Verification items for the finished model (mm, model axes). A direction names the side the tool comes from. Round coordinates to 2 decimals unless told otherwise and drop trailing zeros. Order: outer loops, then holes, each group sorted by start corner. A loop starts at its lowest first (then second) coordinate and runs counter-clockwise, first axis right, second up. Notation, with made-up numbers: (4.25, -24.75) -> (47.25, -24.75) arc R15 cw to (47.25, 4.25) -> close; hole circle Ø5 at (72.25, 80.25). An arc over 180 degrees is marked (long way). Put each result on its own line as item: value.
```python
from build123d import *

# Parameters (mm, degrees)
BOSS_EXTRUDE1_DEPTH    = 105
SKETCH3_R              = 1.75
CUT_EXTRUDE1_DEPTH     = 15
CUT_EXTRUDE2_START     = -3
CUT_EXTRUDE2_OUTLINE_R = 1.75
CUT_EXTRUDE2_DEPTH     = 3
FILLET1_R              = 1


# Read off the part's stored shape, not the designer's step: Cut-Extrude2
with BuildPart() as part:
    # Sketch1 → Boss-Extrude1 (new body)
    with BuildSketch(Plane.XY):
        with BuildLine():
            ThreePointArc((-43.375, -14.309088021), (-30.875, -19), (-18.375, -14.309088021))
            Line((-18.375, -14.309088021), (-18.375, -3.570714214))
            ThreePointArc((-18.375, -3.570714214), (-30.875, -13), (-43.375, -3.570714214))
            Line((-43.375, -3.570714214), (-43.375, -14.309088021))
        make_face()
    extrude(amount=BOSS_EXTRUDE1_DEPTH)

    # Sketch3 → Cut-Extrude1 (cut)
    with BuildSketch(Plane(origin=(0, 0, 0), x_dir=(-1, 0, 0), z_dir=(0, 0, -1))):
        with Locations((22.271353455, -12.287280664)):
            Circle(SKETCH3_R)
        with Locations((30.875, -15)):
            Circle(SKETCH3_R)
        with Locations((39.478646545, -12.287280664)):
            Circle(SKETCH3_R)
    cut_extrude1 = extrude(amount=-CUT_EXTRUDE1_DEPTH, mode=Mode.SUBTRACT)

    # Cut-Extrude2 outline → Cut-Extrude2 (cut)
    # profile 1 of 3: a face of its own
    with BuildSketch(Plane(origin=(0, 0, 4), x_dir=(-1, 0, 0), z_dir=(0, 0, -1)).offset(CUT_EXTRUDE2_START)):
        with BuildLine():
            Line((20.383772748, -14.983025288), (23.662146428, -15.26984582))
            Line((23.662146428, -15.26984582), (25.93448352, -12.024612131))
            ThreePointArc((25.93448352, -12.024612131), (23.418506327, -10.648976576), (21.265316867, -8.755226444))
            Line((21.265316867, -8.755226444), (18.992979775, -12.000460133))
            Line((18.992979775, -12.000460133), (20.383772748, -14.983025288))
        make_face()
        with Locations((22.271353455, -12.287280664)):
            Circle(CUT_EXTRUDE2_OUTLINE_R, mode=Mode.SUBTRACT)
    # profile 2 of 3: a face of its own
    with BuildSketch(Plane(origin=(0, 0, 4), x_dir=(-1, 0, 0), z_dir=(0, 0, -1)).offset(CUT_EXTRUDE2_START)):
        with BuildLine():
            ThreePointArc((40.484683133, -8.755226444), (38.331493673, -10.648976576), (35.81551648, -12.024612131))
            Line((35.81551648, -12.024612131), (38.087853572, -15.26984582))
            Line((38.087853572, -15.26984582), (41.366227252, -14.983025288))
            Line((41.366227252, -14.983025288), (42.757020225, -12.000460133))
            Line((42.757020225, -12.000460133), (40.484683133, -8.755226444))
        make_face()
        with Locations((39.478646545, -12.287280664)):
            Circle(CUT_EXTRUDE2_OUTLINE_R, mode=Mode.SUBTRACT)
    # profile 3 of 3: a face of its own
    with BuildSketch(Plane(origin=(0, 0, 4), x_dir=(-1, 0, 0), z_dir=(0, 0, -1)).offset(CUT_EXTRUDE2_START)):
        with BuildLine():
            ThreePointArc((33.725, -12.683749446), (30.875, -13), (28.025, -12.683749446))
            Line((28.025, -12.683749446), (28.025, -16.645448267))
            Line((28.025, -16.645448267), (30.875, -18.290896534))
            Line((30.875, -18.290896534), (33.725, -16.645448267))
            Line((33.725, -16.645448267), (33.725, -12.683749446))
        make_face()
        with Locations((30.875, -15)):
            Circle(CUT_EXTRUDE2_OUTLINE_R, mode=Mode.SUBTRACT)
    cut_extrude2 = extrude(amount=CUT_EXTRUDE2_DEPTH, mode=Mode.SUBTRACT)

    # Mirror1: Cut-Extrude1, Cut-Extrude2 across plane
    add(cut_extrude1.mirror(Plane(origin=(0, 0, 52.5), x_dir=(1, 0, 0), z_dir=(0, 0, -1))), mode=Mode.SUBTRACT)
    add(cut_extrude2.mirror(Plane(origin=(0, 0, 52.5), x_dir=(1, 0, 0), z_dir=(0, 0, -1))), mode=Mode.SUBTRACT)

    # Fillet1
    fillet1_edges = [part.edges().sort_by_distance(p)[0] for p in [
        (-18.375, -3.570714214, 52.5),
        (-43.375, -3.570714214, 52.5),
    ]]
    fillet(fillet1_edges, radius=FILLET1_R)


solid = part.part
```
Item 1: Material ranges on line 1 along Z through (x, y) = (-20, -11.75); line 2 along X through (y, z) = (-7.75, 44.5); line 3 along X through (y, z) = (-10.75, 58.5) (3 decimals), recorded low to high.
Geometry check:
line 1: 0 to 4, 7 to 98, 101 to 105
line 2: -43.35 to -41.31, -20.44 to -18.4
line 3: -43.375 to -38.185, -23.565 to -18.375
Item 2: Tool access check on faces 1 (the face through (-41.095, -12.958, 10.944)), 2 (the face through (-23.94, -11.76, 94.06)), 3 (the face through (-32.28, -17.48, 5.52)), 4 (the face through (-39.7, -15.13, 5.52)). Record the directions out of +Z, -Z, +X, -X, +Y, -Y that give a thin tool (end or side, any length) a straight path to the whole face; none if there is none.
Geometry check:
face 1: -Z
face 2: +Z
face 3: +Y
face 4: none
Item 3: Release check for a two-part mould opening along Z. For faces 5 (the face through (-22, -12, 15)), 6 (the face through (-31, -15, 90)), 7 (the face through (-41.095, -12.958, 94.056)), 8 (the face through (-40.01, -14.14, 4)) record: pulls with the +Z half, pulls with the -Z half, needs draft (parallel to the pull), parting line crosses it, or undercut.
Geometry check:
face 5: pulls with the -Z half
face 6: pulls with the +Z half
face 7: needs draft
face 8: undercut
Item 4: Sectioned sample at A-A, the plane x = -30. Record the boundary of the cut face in (y, z), then the cut area to 3 significant figures.
Geometry check:
outline: (-18.98, 0) -> (-16.52, 0) -> (-16.52, 4) -> (-17.79, 4) -> (-17.79, 7) -> (-16.52, 7) -> (-16.52, 15) -> (-13.48, 15) -> (-13.48, 7) -> (-12.97, 7) -> (-12.97, 98) -> (-13.48, 98) -> (-13.48, 90) -> (-16.52, 90) -> (-16.52, 98) -> (-17.79, 98) -> (-17.79, 101) -> (-16.52, 101) -> (-16.52, 105) -> (-18.98, 105) -> close; (-13.48, 0) -> (-12.97, 0) -> (-12.97, 4) -> (-13.48, 4) -> close; (-13.48, 101) -> (-12.97, 101) -> (-12.97, 105) -> (-13.48, 105) -> close
area: 529 mm2
Item 5: Depth check by flat-ended pin: pin 1 Ø1.5 at (x, z) = (-23, 48.5) entering from +Y; pin 2 Ø1 at (x, y) = (-40, -12) entering from -Z; pin 3 Ø1 at (x, z) = (-40.5, 56) entering from -Y. Enter the tip coordinate at first touch or a pass-through.
Geometry check:
pin 1: y = -9.73
pin 2: z = 15
pin 3: y = -16.67
Item 6: Sectioned sample at B-B, the plane z = 18.5. Record the boundary of the cut face in (x, y) (3 decimals), then the cut area to 3 significant figures.
Geometry check:
outline: (-43.375, -14.309) arc R19 ccw to (-18.375, -14.309) -> (-18.375, -7.984) arc R1 ccw to (-20.196, -7.414) arc R13 cw to (-41.554, -7.414) arc R1 ccw to (-43.375, -7.984) -> close
area: 170 mm2
